Input: part model. Units: mm. Frame: model coordinates. Face numbers are marked on the shaded views. A direction names the side the tool comes from. Give positions to 0.01 mm unless a question says otherwise; leave off trailing zeros. Loops run counter-clockwise (first coordinate to the right, second up) from the corner with the lowest first, then second, coordinate; pieces in that order, holes last. Notation, with made-up numbers: M 45.5,41.5 L 101.5,41.5 A19 ccw 101.5,49.5 Z; hole C -24,66 d4. An arc over 180 degrees is marked long. Return JSON: item names as keys, results as strings. Group by question number.
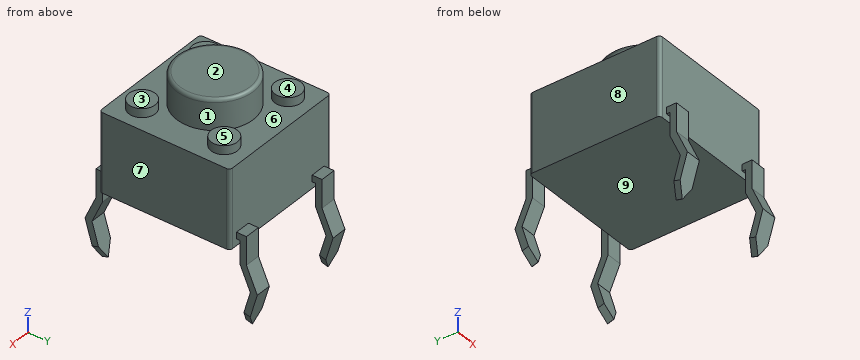
```python
from build123d import *

# Parameters (mm, degrees)
SKETCH2_W                 = 5.99
SKETCH2_H                 = 5.99
BOSS_EXTRUDE1_DEPTH       = 3.6
SKETCH3_R                 = 1.75
BOSS_EXTRUDE2_DEPTH       = 1.4
EXTRUDE_THIN1_DEPTH       = 0.355
CHAMFER2_SIZE             = 0.35
CHAMFER2_SIZE2            = 0.606217783
CHAMFER2_OF_MIRROR1_SIZE2 = 0.35
CHAMFER2_OF_MIRROR1_SIZE  = 0.606217783
FILLET1_R                 = 0.15
SKETCH5_R                 = 0.6
BOSS_EXTRUDE3_DEPTH       = 0.4


# Read off the part's stored shape, not the designer's step: Mirror2
with BuildPart() as part:
    # Sketch2 → Boss-Extrude1 (new body)
    with BuildSketch(Plane.XY):
        with Locations((2.995, 2.995)):
            Rectangle(SKETCH2_W, SKETCH2_H)
    extrude(amount=BOSS_EXTRUDE1_DEPTH)

    # Sketch3 → Boss-Extrude2 (add)
    with BuildSketch(Plane.XY.offset(3.6)):
        with Locations(Location((2.995, 2.995, 0), (0, 0, 180))):
            Circle(SKETCH3_R)
    extrude(amount=BOSS_EXTRUDE2_DEPTH)

    # Sketch4 → Extrude-Thin1 (add, symmetric)
    with BuildSketch(Plane(origin=(5.24, 0, 0), x_dir=(0, 0, -1), z_dir=(1, 0, 0))):
        Polygon((-0.6, 5.99), (-0.6, 6.445), (0.68, 6.445), (1.8, 6.945), (3.5, 6.445), (3.415350103, 6.15719035), (1.821377167, 6.626005919), (0.743923909, 6.145), (-0.3, 6.145), (-0.3, 5.99), align=None)
    extrude_thin1 = extrude(amount=EXTRUDE_THIN1_DEPTH, both=True)

    # Chamfer2
    chamfer2_edges = [part.edges().sort_by_distance(p)[0] for p in [
        (5.595, 6.301095175, -3.457675051),
        (4.885, 6.301095175, -3.457675051),
    ]]
    chamfer2_side = [part.faces().sort_by_distance(p)[0] for p in [
        (5.24, 6.301095175, -3.457675051),
    ]]
    chamfer(chamfer2_edges, length=CHAMFER2_SIZE, length2=CHAMFER2_SIZE2, reference=chamfer2_side[0])

    # Mirror1: Extrude-Thin1 across plane
    add(extrude_thin1.mirror(Plane(origin=(2.995, 0, 0), x_dir=(0, 0, 1), z_dir=(1, 0, 0))))

    # Chamfer2 of Mirror1
    chamfer2_of_mirror1_edges = [part.edges().sort_by_distance(p)[0] for p in [
        (0.395, 6.301095175, -3.457675051),
        (1.105, 6.301095175, -3.457675051),
    ]]
    chamfer(chamfer2_of_mirror1_edges, length=CHAMFER2_OF_MIRROR1_SIZE, length2=CHAMFER2_OF_MIRROR1_SIZE2)

    # Mirror2: part across plane


with BuildPart() as part_1:
    add(part.part)
    add(part.part.mirror(Plane.ZX.offset(2.995)))

    # Fillet1
    fillet1_edges = [part_1.edges().sort_by_distance(p)[0] for p in [
        (4.745, 2.995, 5),
        (0, 5.99, 1.8),
        (5.99, 5.99, 1.8),
        (5.99, 0, 1.8),
        (0, 0, 1.8),
    ]]
    fillet(fillet1_edges, radius=FILLET1_R)

    # Sketch5 → Boss-Extrude3 (add)
    with BuildSketch(Plane.XY.offset(3.6)):
        with Locations(Location((1.105, 4.88, 0), (0, 0, 180))):
            Circle(SKETCH5_R)
        with Locations(Location((4.885, 4.88, 0), (0, 0, 180))):
            Circle(SKETCH5_R)
        with Locations(Location((4.885, 1.11, 0), (0, 0, 180))):
            Circle(SKETCH5_R)
        with Locations(Location((1.105, 1.11, 0), (0, 0, 180))):
            Circle(SKETCH5_R)
    extrude(amount=BOSS_EXTRUDE3_DEPTH)


solid = part_1.part
```
Item 1: Section B-B, the plane z = -1. Return loops of the section in (x, y) (3 decimals).
Item 2: Reachability of the marked faces 1, 2, 3, 4 and 5 from +Z, -Z, +X, -X, +Y, -Y: full face, straight path, thin tool, end or side. Return the list, or none.
Item 3: First-contact query: pin 1 Ø0.5 at (y, z) = (-0.5, -1.5) entering from -X (3 decimals); pin 2 Ø1.8 at (x, y) = (2, 2) entering from -Z; pin 3 Ø0.6 at (x, z) = (5.5, 0) entering from -Y (3 decimals). Flat tips, straight axial feed; report the tip coordinate or a pass-through.
Item 4: Pull-direction query (X, two-part tool) for the marked faces 6, 7, 8 and 9; classes: pulls with the +X half, pulls with the -X half, needs draft (parallel to the pull), parting line crosses it, or undercut.
Item 5: Section C-C, the plane z = 2.25. Return loops of the section in (x, y).
Item 6: Section A-A, the plane y = 4.88. Return loops of the section in (x, z) (3 decimals).
Item 7: Material intervals for line 1 (Z direction, x = 5.3, y = 5); line 2 (Y direction, x = 1.25, z = 0.5); line 3 (Z direction, x = 2.2, y = 1), sorted ascending. Write a range as from..to.
Answer below:
{
 "1": {"outline": "M 0.395,-0.598 L 1.105,-0.598 L 1.105,-0.269 L 0.395,-0.269 Z; M 0.395,6.259 L 1.105,6.259 L 1.105,6.588 L 0.395,6.588 Z; M 4.885,-0.598 L 5.595,-0.598 L 5.595,-0.269 L 4.885,-0.269 Z; M 4.885,6.259 L 5.595,6.259 L 5.595,6.588 L 4.885,6.588 Z"},
 "2": {"face 1": "+Z", "face 2": "+Z, +X, -X, +Y, -Y", "face 3": "+Z, +X, -Y", "face 4": "+Z, -X, +Y", "face 5": "+Z, +X, +Y"},
 "3": {"pin 1": "x = 0.395", "pin 2": "z = 0", "pin 3": "y = -0.455"},
 "4": {"face 6": "undercut", "face 7": "pulls with the +X half", "face 8": "pulls with the -X half", "face 9": "needs draft"},
 "5": {"outline": "M 0,0.15 A0.15 ccw 0.15,0 L 5.84,0 A0.15 ccw 5.99,0.15 L 5.99,5.84 A0.15 ccw 5.84,5.99 L 0.15,5.99 A0.15 ccw 0,5.84 Z"},
 "6": {"outline": "M 0,0 L 5.99,0 L 5.99,3.6 L 5.485,3.6 L 5.485,4 L 4.285,4 L 4.285,3.6 L 1.705,3.6 L 1.705,4 L 0.505,4 L 0.505,3.6 L 0,3.6 Z"},
 "7": {"line 1": "0..4", "line 2": "0..5.99", "line 3": "0..3.6"}
}
